The listing builds one solid part. Answer for the finished solid, in the listing's coordinates (mm). A direction names the side the tool comes from. Give positions to 0.01 mm unless a question says otherwise; leave off trailing zeros. Write each loop counter-clockwise with the first axis right and the second up, starting at its lowest first coordinate (ties: lowest second). Pieces come first, ordered by that corner, then holes. Notation, with made-up numbers: (-34.75, 1) - (-2.75, 1) arc R14 cw to (-2.75, 25) - close; hole circle Ø10 at (85.5, -38.5). An arc over 180 degrees is marked (long way). Use a Markdown table: item, result. Add a question column.
from build123d import *

# Parameters (mm, degrees)
EXTRUDE_1_DEPTH          = 7
CUT_EXTRUDE_1_DEPTH      = 140.270420406
CUT_EXTRUDE_1_DEPTH_BACK = 140.270420406
CUT_EXTRUDE_2_DEPTH      = 5
SKETCH_12_R              = 1.45
CUT_EXTRUDE_3_DEPTH      = 140.270420406
SKETCH_14_R              = 12
CUT_EXTRUDE_4_DEPTH      = 140.270420406
SKETCH_15_R              = 3.5
CUT_EXTRUDE_5_DEPTH      = 10
SKETCH_16_R              = 2.8
CUT_EXTRUDE_6_DEPTH      = 3
PATTERN_CIRCULAR_1_COUNT = 6


with BuildPart() as part:
    # Sketch 2 → Extrude 1 (new body)
    with BuildSketch(Plane.XY):
        with BuildLine():
            Line((1.428, 20.951391744), (125.85, 12.471066514))
            ThreePointArc((125.85, 12.471066514), (137.5, 0), (125.85, -12.471066514))
            Line((125.85, -12.471066514), (1.428, -20.951391744))
            ThreePointArc((1.428, -20.951391744), (-21, 0), (1.428, 20.951391744))
        make_face()
    extrude(amount=EXTRUDE_1_DEPTH)

    # Sketch 3 → Cut-Extrude 1 (cut, two sides: drawn at the far end of the back side and taken through both)
    with BuildSketch(Plane.XY.offset(7).offset(-CUT_EXTRUDE_1_DEPTH_BACK)):
        Polygon((44.657987472, 12.993332243), (14.657987472, -15.038065143), (44.657987472, -12.993332243), align=None)
        Polygon((94.699739521, 9.58259835), (99.519663952, -9.254083082), (111.519663952, 8.436189922), align=None)
        Polygon((89.447040438, 9.940610571), (59.071666369, -12.010928128), (94.447040438, -9.599821755), align=None)
        with BuildLine():
            Line((37.832309087, 13.458555215), (14.657987472, 15.038065143))
            ThreePointArc((14.657987472, 15.038065143), (19.784577979, 7.04063024), (20.86269223, -2.397513905))
            Line((20.86269223, -2.397513905), (37.832309087, 13.458555215))
        make_face()
        Polygon((49.646414078, 12.653332243), (49.646414078, -12.653332243), (81.646414078, 10.472283817), align=None)
    extrude(amount=CUT_EXTRUDE_1_DEPTH + CUT_EXTRUDE_1_DEPTH_BACK, mode=Mode.SUBTRACT)

    # Sketch 7 → Cut-Extrude 2 (cut)
    with BuildSketch(Plane.XY.offset(7)):
        Polygon((127.879739572, 5), (122.120260428, 5), (119.23, 0), (122.120260428, -5), (127.879739572, -5), (130.77, 0), align=None)
    extrude(amount=-CUT_EXTRUDE_2_DEPTH, mode=Mode.SUBTRACT)

    # Sketch 12 → Cut-Extrude 3 (cut, through all)
    with BuildSketch(Plane.XY.offset(7)):
        with Locations((0, 15)):
            Circle(SKETCH_12_R)
        with Locations((12.990381057, 7.5)):
            Circle(SKETCH_12_R)
        with Locations((12.990381057, -7.5)):
            Circle(SKETCH_12_R)
        with Locations((0, -15)):
            Circle(SKETCH_12_R)
        with Locations((-12.990381057, -7.5)):
            Circle(SKETCH_12_R)
        with Locations((-12.990381057, 7.5)):
            Circle(SKETCH_12_R)
    extrude(amount=-CUT_EXTRUDE_3_DEPTH, mode=Mode.SUBTRACT)

    # Sketch 14 → Cut-Extrude 4 (cut, through all)
    with BuildSketch(Plane.XY.offset(7)):
        Circle(SKETCH_14_R)
    extrude(amount=-CUT_EXTRUDE_4_DEPTH, mode=Mode.SUBTRACT)

    # Sketch 15 → Cut-Extrude 5 (cut)
    with BuildSketch(Plane(origin=(0, 0, 0), x_dir=(-1, 0, 0), z_dir=(0, 0, -1))):
        with Locations((-125, 0)):
            Circle(SKETCH_15_R)
    extrude(amount=-CUT_EXTRUDE_5_DEPTH, mode=Mode.SUBTRACT)

    # Sketch 16 → Cut-Extrude 6 (cut)
    with BuildSketch(Plane(origin=(0, 0, 0), x_dir=(-1, 0, 0), z_dir=(0, 0, -1))):
        with Locations((0, 15)):
            Circle(SKETCH_16_R)
    cut_extrude_6 = extrude(amount=-CUT_EXTRUDE_6_DEPTH, mode=Mode.SUBTRACT)

    # Pattern Circular 1: Cut-Extrude 6 ×6 about axis
    pattern_circular_1_axis = Axis((0, 0, 0), (0, 0, 1))
    for i in range(1, PATTERN_CIRCULAR_1_COUNT):
        add(cut_extrude_6.rotate(pattern_circular_1_axis, i * 360 / PATTERN_CIRCULAR_1_COUNT), mode=Mode.SUBTRACT)


solid = part.part
1. The part is cut by section D-D (x = 124.5). Give the vertices of the cut face in (y, z), and give its area (3 significant figures).
2. Given P1, Ø7.5, axis at x = 0, y = -15, coming from the -Z side; P2, Ø3, axis at x = -12, y = 7.5, coming from the -Z side; P3, Ø4, axis at x = 126, z = 4, coming from the -Y side; P4, Ø2, axis at y = -6, z = 5, coming from the +X side, each flat-ended and moving along its own axis, determine where each tip first touches the part or whether it passes through.
3. The part is cut by section B-B (x = 0). Give the vertices of the cut face in (y, z), and give its area (3 significant figures).
4. The part is cut by section C-C (x = 23). Give the vertices of the cut face in (y, z).
5. The part is cut by section A-A (z = 5). Count the separate pieces of the cut face and the enclosed holes in it, and give its area (3 significant figures).
6. For a pull along X with two mould halves and no side action, classify faces 1 (the flat face through (64.51, -16.65, 3.45)), 2 (the flat face through (29.868, -0.826, 3.451)) as released by +X, released by -X, zero draft, split by the parting line, or undercut.
7. Which of the six approach directions +Z, -Z, +X, -X, +Y, -Y give full straight-line access (tool end or side, diameter ignored) to faces 3 (the cylindrical face through (15.054, -5.608, 1.479)), 4 (the flat face through (26.407, 14.237, 3.451)), 5 (the flat face through (120.65, -2.46, 4.54))?
8. Consider L1, parallel to Y at x = 0, z = 4.4; L2, parallel to Y at x = 0, z = 0.7; L3, parallel to Y at x = 26.5, z = 4. Determine where each line is inside the solid, lowest interval first. Write a range as [from, to].
Check values:
| question | item | result |
|---|---|---|
| 1 | outline | (-12.56, 0) - (-3.46, 0) - (-3.46, 2) - (-5, 2) - (-5, 7) - (-12.56, 7) - close; (3.46, 0) - (12.56, 0) - (12.56, 7) - (5, 7) - (5, 2) - (3.46, 2) - close |
| 1 | area | 112 mm2 |
| 2 | P1 | stops at z = 0 |
| 2 | P2 | stops at z = 3 |
| 2 | P3 | stops at y = -12.6 |
| 2 | P4 | stops at x = 136.46 |
| 3 | outline | (-21, 0) - (-17.8, 0) - (-17.8, 3) - (-16.45, 3) - (-16.45, 7) - (-21, 7) - close; (-13.55, 3) - (-12.2, 3) - (-12.2, 0) - (-12, 0) - (-12, 7) - (-13.55, 7) - close; (12, 0) - (12.2, 0) - (12.2, 3) - (13.55, 3) - (13.55, 7) - (12, 7) - close; (16.45, 3) - (17.8, 3) - (17.8, 0) - (21, 0) - (21, 7) - (16.45, 7) - close |
| 3 | area | 69.2 mm2 |
| 4 | outline | (-19.48, 0) - (-14.47, 0) - (-14.47, 7) - (-19.48, 7) - close; (-7.24, 0) - (-0.4, 0) - (-0.4, 7) - (-7.24, 7) - close; (14.47, 0) - (19.48, 0) - (19.48, 7) - (14.47, 7) - close |
| 5 | separate pieces | 1 |
| 5 | enclosed holes | 13 |
| 5 | area | 3,080 mm2 |
| 6 | face 1 | released by +X |
| 6 | face 2 | undercut |
| 7 | face 3 | -Z |
| 7 | face 4 | +Z, -Z |
| 7 | face 5 | +Z |
| 8 | L1 | y = [-21, -16.45], [-13.55, -12], [12, 13.55], [16.45, 21] |
| 8 | L2 | y = [-21, -17.8], [-12.2, -12], [12, 12.2], [17.8, 21] |
| 8 | L3 | y = [-19.24, -14.23], [-3.97, 2.87], [14.23, 19.24] |
